```python
from build123d import *

# Parameters (mm, degrees)
BOSS_EXTRU_1_DEPTH      = 2.5
ESQUISSE2_R             = 1.6
ENL_V_MAT_EXTRU_1_DEPTH = 3.5
BOSS_EXTRU_2_DEPTH      = 9.5
CONG_2_R                = 1
CONG_1_R                = 2.5
ESQUISSE4_R             = 1.6
ENL_V_MAT_EXTRU_2_DEPTH = 13


with BuildPart() as part:
    # Esquisse1 → Boss.-Extru.1 (new body)
    with BuildSketch(Plane.XY):
        Polygon((-6.4, 0), (6.11755814, 0), (6.4, 0), (56, 75.87), (40.7, 75.87), (7.443745881, 25), (-7.443745881, 25), (-40.7, 75.87), (-56, 75.87), align=None)
    extrude(amount=BOSS_EXTRU_1_DEPTH)

    # Esquisse2 → Enlèv. mat.-Extru.1 (cut, through all)
    with BuildSketch(Plane.XY.offset(2.5)):
        with Locations((0, 4.7)):
            Circle(ESQUISSE2_R)
    extrude(amount=-ENL_V_MAT_EXTRU_1_DEPTH, mode=Mode.SUBTRACT)

    # Esquisse3 → Boss.-Extru.2 (add)
    with BuildSketch(Plane(origin=(0, 0, 0), x_dir=(-1, 0, 0), z_dir=(0, 0, -1))):
        Polygon((-35.470001318, 67.87), (-7.443745881, 25), (7.443745881, 25), (35.470001318, 67.87), (37.859468913, 67.87), (8.525713806, 23), (-8.525713806, 23), (-37.859468913, 67.87), align=None)
    extrude(amount=BOSS_EXTRU_2_DEPTH)

    # Congé2
    cong_2_edges = [part.edges().sort_by_distance(p)[0] for p in [
        (37.859468913, 67.87, -4.75),
        (-37.859468913, 67.87, -4.75),
    ]]
    fillet(cong_2_edges, radius=CONG_2_R)

    # Congé1
    cong_1_edges = [part.edges().sort_by_distance(p)[0] for p in [
        (56, 75.87, 1.25),
        (6.4, 0, 1.25),
        (-6.4, 0, 1.25),
        (-56, 75.87, 1.25),
        (-40.7, 75.87, 1.25),
        (-7.443745881, 25, -3.5),
        (7.443745881, 25, -3.5),
        (40.7, 75.87, 1.25),
    ]]
    fillet(cong_1_edges, radius=CONG_1_R)

    # Esquisse4 → Enlèv. mat.-Extru.2 (cut, through all)
    with BuildSketch(Plane.XY.offset(2.5)):
        with Locations((47.647073462, 72.644280098)):
            Circle(ESQUISSE4_R)
        with Locations((-47.647073462, 72.644280098)):
            Circle(ESQUISSE4_R)
    extrude(amount=-ENL_V_MAT_EXTRU_2_DEPTH, mode=Mode.SUBTRACT)


solid = part.part
```
Check sheet for the modelled part. Datum: model origin and axes. Units: mm. A direction names the side the tool comes from. Round coordinates to 2 decimals unless told otherwise and drop trailing zeros. Loops run counter-clockwise (first coordinate to the right, second up) from the corner with the lowest first, then second, coordinate; pieces in that order, holes last. Notation, with made-up numbers: (-16, 23) - (22, 23) arc R28 ccw to (22, 42) - close; hole circle Ø7 at (-24.5, 2). An arc over 180 degrees is marked (long way). Answer as a JSON object with one key per item and string values. Group by question number.
Q1. Scan lines: line 1 along Y through (x, z) = (0, 1.5); line 2 along Z through (x, y) = (4, 15.5); line 3 along X through (y, z) = (65, -5.5). Record each from-to range of solid material in increasing order. Write a range as [from, to].
Q2. Sectioned sample at A-A, the plane x = 0. Enter the section's corners in (y, z), plus the area to 3 significant figures.
Q3. Sectioned sample at C-C, the plane z = -7.25. Enter the section's corners in (x, y).
Q4. Sectioned sample at B-B, the plane y = 37. Enter the section's corners in (x, z), plus the area to 3 significant figures.
Q5. Mould release check, pull along Y, two halves, no side actions. Record for faces 4 (the face through (-30.63, 37.06, 1.23)), 5 (the face through (47, 75.87, 1)), 6 (the face through (47.3, 71.082, 1.268)): released by +Y, released by -Y, zero draft, split by the parting line, or undercut.
Q6. Set-up check for faces 1 (the face through (-12, 30, 2.5)), 2 (the face through (0, 23, -5)), 3 (the face through (0, 25, -3)): record each of +Z, -Z, +X, -X, +Y, -Y from which the full face is reachable in a straight line by a thin tool's end or side.
Q7. Gauge pin test, flat ends, axial feed: P1, Ø4, axis at x = -47.65, y = 72.64, coming from the +Z side; P2, Ø5, axis at y = 61.5, z = -6, coming from the +X side; P3, Ø3.5, axis at x = 47.65, y = 72.64, coming from the -Z side; P4, Ø3, axis at x = 0, y = 4.7, coming from the +Z side. Record the tip position at first contact, or that the pin passes through.
Q8. Sectioned sample at D-D, the plane y = 4.7. Enter the section's corners in (x, z), plus the area to 3 significant figures.
Solution:
{
 "1": {"line 1": "y = [0, 3.1], [6.3, 25]", "line 2": "z = [0, 2.5]", "line 3": "x = [-35.98, -33.59], [33.59, 35.98]"},
 "2": {"outline": "(0, 0) - (3.1, 0) - (3.1, 2.5) - (0, 2.5) - close; (6.3, 0) - (23, 0) - (23, -9.5) - (25, -9.5) - (25, 2.5) - (6.3, 2.5) - close", "area": "73.5 mm²"},
 "3": {"outline": "(-36.85, 66.32) - (-8.53, 23) - (8.53, 23) - (36.85, 66.32) arc R1 ccw to (36.01, 67.87) - (35.47, 67.87) - (8.18, 26.13) arc R2.5 cw to (6.09, 25) - (-6.09, 25) arc R2.5 cw to (-8.18, 26.13) - (-35.47, 67.87) - (-36.01, 67.87) arc R1 ccw to start"},
 "4": {"outline": "(-30.59, 0) - (-17.68, 0) - (-17.68, -9.5) - (-15.29, -9.5) - (-15.29, 2.5) - (-30.59, 2.5) - close; (15.29, -9.5) - (17.68, -9.5) - (17.68, 0) - (30.59, 0) - (30.59, 2.5) - (15.29, 2.5) - close", "area": "122 mm²"},
 "5": {"face 4": "released by -Y", "face 5": "released by +Y", "face 6": "undercut"},
 "6": {"face 1": "+Z, +X, -X, +Y, -Y", "face 2": "-Z, +X, -X, -Y", "face 3": "+Z, -Z, +Y"},
 "7": {"P1": "stops at z = 2.5", "P2": "stops at x = 35.33", "P3": "stops at z = 0", "P4": "passes through"},
 "8": {"outline": "(-9.47, 0) - (-1.6, 0) - (-1.6, 2.5) - (-9.47, 2.5) - close; (1.6, 0) - (9.47, 0) - (9.47, 2.5) - (1.6, 2.5) - close", "area": "39.4 mm²"}
}
